from build123d import *

# Parameters (mm, degrees)
SKETCH_1_R               = 15
SKETCH_1_R_2             = 5
EXTRUDE_1_DEPTH          = 8
SKETCH_2_W               = 4
SKETCH_2_H               = 4
CUT_EXTRUDE_1_DEPTH      = 23.671568098
SKETCH_3_W               = 2
SKETCH_3_H               = 20
CUT_EXTRUDE_2_DEPTH      = 23.671568098
CUT_EXTRUDE_3_DEPTH      = 23.671568098
CUT_EXTRUDE_3_DEPTH_BACK = 23.671568098
SKETCH_4_R               = 1.7
SKETCH_5_R               = 3
CUT_EXTRUDE_4_DEPTH      = 10
SKETCH_6_R               = 1.5
CUT_EXTRUDE_5_DEPTH      = 23.671568265
CHAMFER_1_SIZE           = 0.5


with BuildPart() as part:
    # 草图1 → 凸台-拉伸1 (new body)
    with BuildSketch(Plane(origin=(0, 0, 0), x_dir=(1, 0, 0), z_dir=(0, 1, 0))):
        with Locations(Location((0, 0, 0), (0, 0, 270))):
            Circle(SKETCH_1_R)
        with Locations(Location((0, 0, 0), (0, 0, 270))):
            Circle(SKETCH_1_R_2, mode=Mode.SUBTRACT)
    extrude(amount=EXTRUDE_1_DEPTH)

    # 草图2 → 切除-拉伸1 (cut, through all)
    with BuildSketch(Plane(origin=(0, 8, 0), x_dir=(1, 0, 0), z_dir=(0, 1, 0))):
        with Locations((0, 6)):
            Rectangle(SKETCH_2_W, SKETCH_2_H)
    extrude(amount=-CUT_EXTRUDE_1_DEPTH, mode=Mode.SUBTRACT)

    # 草图3 → 切除-拉伸2 (cut, through all)
    with BuildSketch(Plane(origin=(0, 8, 0), x_dir=(1, 0, 0), z_dir=(0, 1, 0))):
        with Locations((0, -5)):
            Rectangle(SKETCH_3_W, SKETCH_3_H)
    extrude(amount=-CUT_EXTRUDE_2_DEPTH, mode=Mode.SUBTRACT)

    # 草图4 → 切除-拉伸3 (cut, two sides: drawn at the far end of the back side and taken through both)
    with BuildSketch(Plane(origin=(0, 0, 0), x_dir=(0, 0, -1), z_dir=(1, 0, 0)).offset(-CUT_EXTRUDE_3_DEPTH_BACK)):
        with Locations((-10.966629547, 4)):
            Circle(SKETCH_4_R)
    extrude(amount=CUT_EXTRUDE_3_DEPTH + CUT_EXTRUDE_3_DEPTH_BACK, mode=Mode.SUBTRACT)

    # 草图5 → 切除-拉伸4 (cut)
    with BuildSketch(Plane(origin=(15, 0, 0), x_dir=(0, 0, -1), z_dir=(1, 0, 0))):
        with Locations((-10.966629547, 4)):
            Circle(SKETCH_5_R)
    cut_extrude_4 = extrude(amount=-CUT_EXTRUDE_4_DEPTH, mode=Mode.SUBTRACT)

    # 镜向1: 切除-拉伸4 across plane
    add(cut_extrude_4.mirror(Plane(origin=(0, 0, 0), x_dir=(0, 0, 1), z_dir=(1, 0, 0))), mode=Mode.SUBTRACT)

    # 草图6 → 切除-拉伸5 (cut, through all)
    with BuildSketch(Plane(origin=(0, 8, 0), x_dir=(1, 0, 0), z_dir=(0, 1, 0))):
        with Locations(Location((10, 0, 0), (0, 0, 270))):
            Circle(SKETCH_6_R)
        with Locations(Location((-10, 0, 0), (0, 0, 90))):
            Circle(SKETCH_6_R)
    extrude(amount=-CUT_EXTRUDE_5_DEPTH, mode=Mode.SUBTRACT)

    # 倒角1
    chamfer_1_edges = [part.edges().sort_by_distance(p)[0] for p in [
        (-4.972421157, 0, 0.524430968),
        (4.972421157, 0, 0.524430968),
        (4.972421157, 8, 0.524430968),
        (0, 8, -15),
        (0, 0, -15),
        (10, 0, -1.5),
        (10, 8, -1.5),
        (-10, 0, 1.5),
        (-10, 8, 1.5),
        (-4.972421157, 8, 0.524430968),
    ]]
    chamfer(chamfer_1_edges, length=CHAMFER_1_SIZE)


solid = part.part
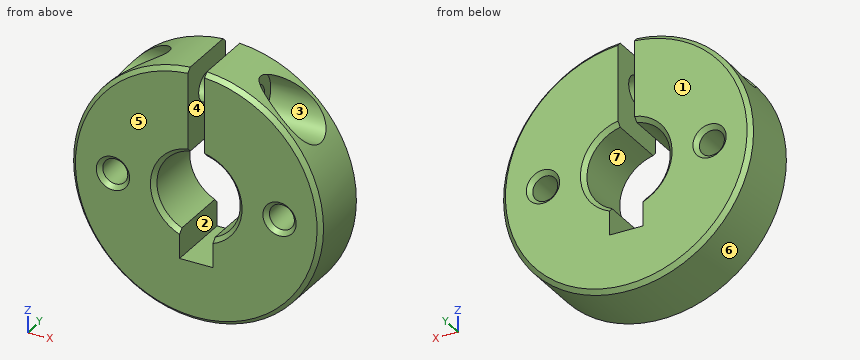
Source: CAD feature listing. Evaluate the final solid. Frame: model axes, mm. Face numbers are marked on the shaded views. A direction names the side the tool comes from. Give positions to 0.01 mm unless a question says otherwise; leave off trailing zeros. Order: outer loops, then holes, each group sorted by start corner. A loop starts at its lowest first (then second) coordinate and runs counter-clockwise, first axis right, second up. Notation, with made-up numbers: (71.5, -31) -> (111.5, -31) arc R23 cw to (111.5, -19) -> close; hole circle Ø11 at (-32.75, 3). An arc over 180 degrees is marked (long way). Write item = value, one per line.
Q1. Pin query (flat end, axial travel): pin 1 (2.5 mm diameter, centred on x = 10, z = 0, fed in from +Y); pin 2 (1.5 mm diameter, centred on x = -11.5, y = 6.5, fed in from -Z); pin 3 (3 mm diameter, centred on x = 11.5, y = 3.5, fed in from +Z); pin 4 (4 mm diameter, centred on y = 5.5, z = -6, fed in from +X). Return the tip coordinate at first contact, or that it passes through.
Data:
pin_1 = through
pin_2 = -10.46
pin_3 = 8.73
pin_4 = 14.46
Q2. Pull-direction query (X, two-part tool) for the marked faces 5, 6 and 7; classes: released by +X, released by -X, zero draft, split by the parting line, or undercut.
Data:
face_5 = zero draft
face_6 = split by the parting line
face_7 = undercut
Q3. Set-up query: the marked faces 1, 2, 3 and 4. Return all of +Z, -Z, +X, -X, +Y, -Y with unobstructed straight access to the full face (end or side cutting, diameter ignored); none if empty.
Data:
face_1 = +Z, -Z, +X, -X, +Y
face_2 = +Y, -Y
face_3 = +X
face_4 = +Z, +Y, -Y
Q4. Cut plane C-C, the plane z = 12.25. State how many separate pieces and enclosed holes the cut face has, and give its area (3 significant figures).
Data:
separate_pieces = 4
enclosed_holes = 0
area = 64.1 mm^2
Q5. Cut plane A-A, the plane y = 4. Output: boundary loops of the cut face in (x, z), and give its area (3 significant figures).
Data:
outline = (-12.71, 7.97) arc R15 ccw (long way) to (12.71, 7.97) -> (5, 7.97) -> (5, 9.27) -> (1, 9.27) -> (1, 4.9) arc R5 cw to (2, -4.58) -> (2, -8) -> (-2, -8) -> (-2, -4.58) arc R5 cw to (-1, 4.9) -> (-1, 9.27) -> (-5, 9.27) -> (-5, 7.97) -> close; (-5.47, 13.97) -> (-5, 13.97) -> (-5, 12.67) -> (-1, 12.67) -> (-1, 14.97) arc R15 ccw to start; (1, 12.67) -> (5, 12.67) -> (5, 13.97) -> (5.47, 13.97) arc R15 ccw to (1, 14.97) -> close; hole circle Ø3 at (-10, 0); hole circle Ø3 at (10, 0)
area = 496 mm^2
Q6. Cut plane B-B, the plane x = 0. Output: boundary loops of the cut face in (y, z).
Data:
outline = (0, -14.5) -> (0.5, -15) -> (7.5, -15) -> (8, -14.5) -> (8, -8) -> (0, -8) -> close
Q7. Material intervals for line 1 (X direction, y = 7.75, z = -1.5); line 2 (X direction, y = 1.25, z = -1); line 3 (Z direction, x = 4, y = 4), sorted ascending. Write a range as from..to.
Data:
line_1 = -14.67..-10.9, -9.1..-5.03, 5.03..9.1, 10.9..14.67
line_2 = -14.97..-11.12, -8.88..-4.9, 4.9..8.88, 11.12..14.97
line_3 = -14.46..-3, 3..9.27, 12.67..14.46
